from build123d import *

# Parameters (mm, degrees)
F0_W     = 190.5
F0_H     = 114.3
F0_W_2   = 168.275
F0_H_2   = 88.9
F1_DEPTH = 76.2
F2_W     = 76.2
F2_H     = 76.2
F3_DEPTH = 190.5
F4_R     = 9.525
F5_DEPTH = 190.5


with BuildPart() as f1:
    # F0 (on Top) → F1 (new body)
    with BuildSketch(Plane.XY):
        Rectangle(F0_W, F0_H)
        Rectangle(F0_W_2, F0_H_2, mode=Mode.SUBTRACT)
    extrude(amount=F1_DEPTH)

    # F2 (on face) → F3 (cut, symmetric)
    with BuildSketch(Plane.XZ.offset(57.15)):
        with Locations((0, 76.2)):
            Rectangle(F2_W, F2_H)
    extrude(amount=F3_DEPTH, both=True, mode=Mode.SUBTRACT)

    # F4 (on face) → F5 (cut, symmetric)
    with BuildSketch(Plane.YZ.offset(95.25)):
        with Locations((0, 38.1)):
            Circle(F4_R)
    extrude(amount=F5_DEPTH, both=True, mode=Mode.SUBTRACT)


solid = f1.part
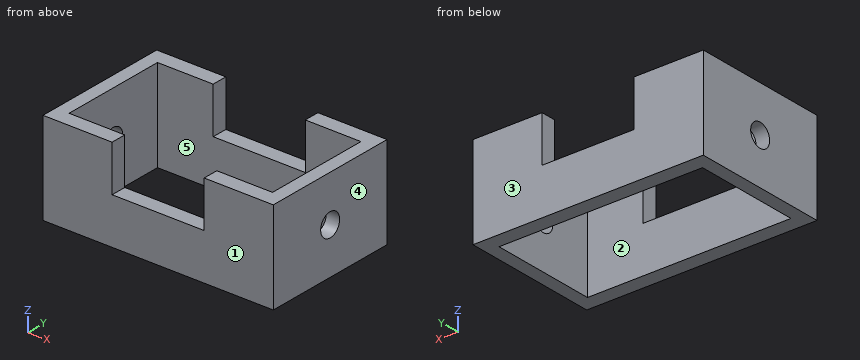
Model file for the job. Use its own axes, mm. Face numbers are marked on the shaded views. A direction names the side the tool comes from. Coordinates: 2 decimals unless noted, no trailing zeros. Write each loop counter-clockwise with the first axis right and the second up, starting at its lowest first coordinate (ties: lowest second). Pieces come first, ordered by that corner, then holes. Notation, with made-up numbers: (-5.75, 86.25) - (20.25, 86.25) arc R9 cw to (20.25, 103.25) - close; hole circle Ø2 at (-26, -35.75). An arc over 180 degrees is marked (long way). Write each question's results on one line, items separated by ' | '. Start each with the question number.
1) Probe line 1 along Y through (x, z) = (-45, 17); line 2 along X through (y, z) = (-26, 14.5). List the from-to ranges inside material, lowest first. Write a range as from..to.
2) 3-axis set-ups, long thin cutter, end or side, ignore diameter. For the marked faces 4 and 5: which of +Z, -Z, +X, -X, +Y, -Y reach the whole face in a straight line?
3) Flat gauge pin, fed straight in: P1, Ø14, axis at x = 18, y = 53.5, coming from the +Z side. Where does the tip first touch, or does it go through?
4) Cut at C-C (x = -53). Write the cut outline in (y, z).
5) Cut at D-D (y = 40). Write the cut outline in (x, z), then the cut area to 3 significant figures.
6) Cut at B-B (y = 0). Count the separate pieces of the cut face and the enclosed holes in it, then the cut area to 3 significant figures.
7) Mould opens along Y. For the marked faces 1, 2 and 3 say: pulls with the +Y half, pulls with the -Y half, needs draft (parallel to the pull), parting line crosses it, or undercut.
8) Cut at A-A (z = 59). Write the cut outline in (x, y).
Returned:
1) line 1: -57.15..-44.45, 44.45..57.15 | line 2: -95.25..-84.14, 84.14..95.25
2) face 4: +Z, -Z, +X, +Y, -Y | face 5: +Z, -Z
3) P1: z = 38.1
4) outline: (-57.15, 0) - (-44.45, 0) - (-44.45, 76.2) - (-57.15, 76.2) - close; (44.45, 0) - (57.15, 0) - (57.15, 76.2) - (44.45, 76.2) - close
5) outline: (-95.25, 0) - (-84.14, 0) - (-84.14, 76.2) - (-95.25, 76.2) - close; (84.14, 0) - (95.25, 0) - (95.25, 76.2) - (84.14, 76.2) - close | area: 1,690 mm^2
6) separate pieces: 4 | enclosed holes: 0 | area: 1,270 mm^2
7) face 1: pulls with the -Y half | face 2: undercut | face 3: pulls with the +Y half
8) outline: (-95.25, -57.15) - (-38.1, -57.15) - (-38.1, -44.45) - (-84.14, -44.45) - (-84.14, 44.45) - (-38.1, 44.45) - (-38.1, 57.15) - (-95.25, 57.15) - close; (38.1, -57.15) - (95.25, -57.15) - (95.25, 57.15) - (38.1, 57.15) - (38.1, 44.45) - (84.14, 44.45) - (84.14, -44.45) - (38.1, -44.45) - close
